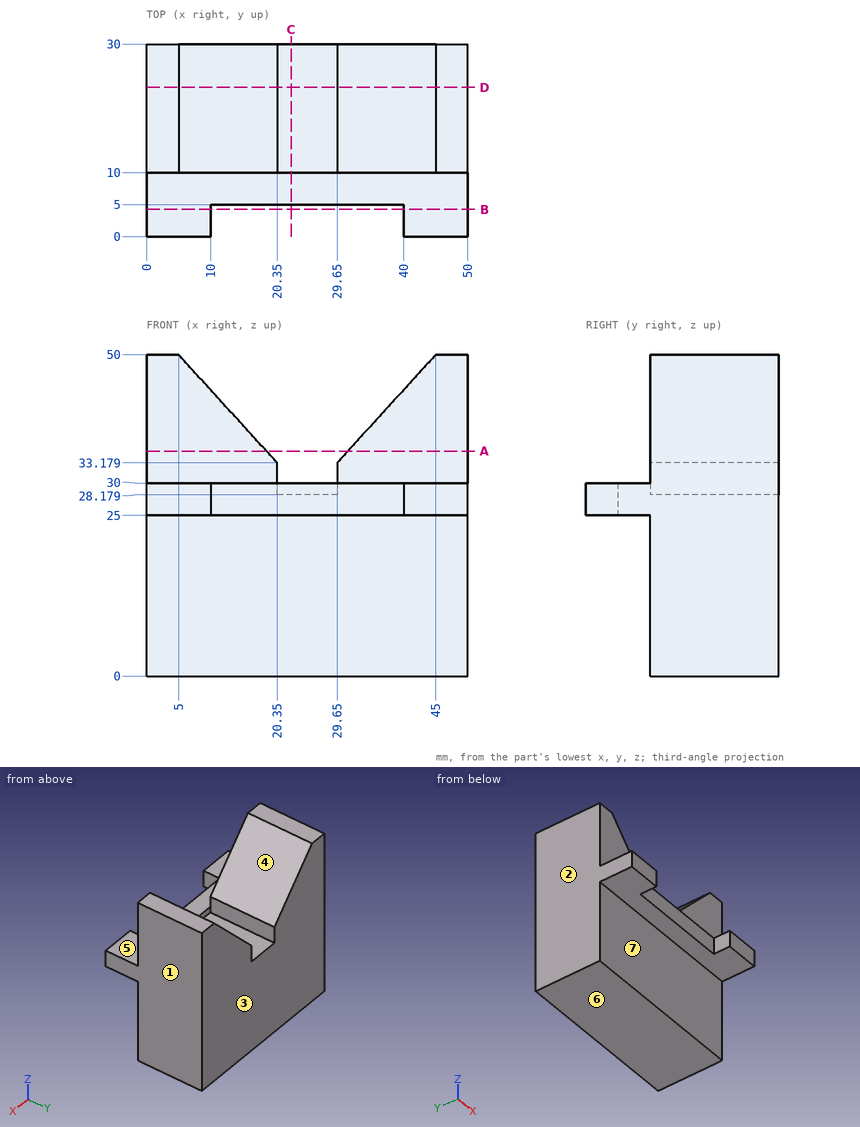
Design review of the part shown in the three views and the two pictorial views. Dimensions are in mm from the part's minimum x, y and z. A direction names the side the tool comes from. Round coordinates to 2 decimals unless told otherwise and drop trailing zeros. Loops run counter-clockwise (first coordinate to the right, second up) from the corner with the lowest first, then second, coordinate; pieces in that order, holes last. Notation, with made-up numbers: M -27.75,29.5 L -19.75,29.5 A14 cw -19.75,35.5 Z; hole C 61,-14 d4. An arc over 180 degrees is marked long. Write item = value, one per line.
Item 1: Take a section at C-C on x = 22.5. Write out the cut boundary in (y, z).
Return value:
outline = M 5,25 L 10,25 L 10,0 L 30,0 L 30,28.18 L 10,28.18 L 10,30 L 5,30 Z
Item 2: Machinability: for the marked faces 5, 6 and 7, which of the approach directions +Z, -Z, +X, -X, +Y, -Y give a long, thin tool a straight path to every point of the face, cutting with its end or side? Answer none if there is none.
Return value:
face_5 = +Z, +X, -X, -Y
face_6 = -Z, +X, -X, +Y, -Y
face_7 = -Z, +X, -X, -Y
Item 3: Take a section at D-D on y = 23.25. Write out the cut boundary in (x, z), then the cut area to 3 significant figures.
Return value:
outline = M 0,0 L 50,0 L 50,50 L 45,50 L 29.65,33.18 L 29.65,28.18 L 20.35,28.18 L 20.35,33.18 L 5,50 L 0,50 Z
area = 2,040 mm2
Item 4: Take a section at B-B on y = 4.25. Write out the cut boundary in (x, z), then the cut area to 3 significant figures.
Return value:
outline = M 0,25 L 10,25 L 10,30 L 0,30 Z; M 40,25 L 50,25 L 50,30 L 40,30 Z
area = 100 mm2
Item 5: Take a section at A-A on z = 35. Write out the cut boundary in (x, y).
Return value:
outline = M 0,10 L 18.69,10 L 18.69,30 L 0,30 Z; M 31.31,10 L 50,10 L 50,30 L 31.31,30 Z
Item 6: Insertion check: P1, Ø2.5, axis at x = 21.5, z = 28, coming from the -Y side; P2, Ø0.5, axis at x = 23, z = 29.5, coming from the +Y side; P3, Ø5, axis at x = 23, y = 5.5, coming from the -Z side; P4, Ø4, axis at y = 16.5, z = 30, coming from the -X side. Each pin has a flat end and moves straight along its axis. Give the tip position at first contact, or say it passes through.
Return value:
P1 = 5
P2 = 10
P3 = 25
P4 = 0
Item 7: The part is to be moulded in two halves that separate along X. For the marked faces 1, 2, 3 and 4, say which applies: released by +X, released by -X, zero draft, split by the parting line, or undercut.
Return value:
face_1 = released by +X
face_2 = released by -X
face_3 = zero draft
face_4 = undercut
Item 8: For line 1 (X direction, y = 22.5, z = 30.5); line 2 (Z direction, x = 2.5, y = 5.25); line 3 (Y direction, x = 19.5, z = 17), list the stretches that pass through material, from the lowest coordinate up. Write a range as [from, to].
Return value:
line_1 = [0, 20.35], [29.65, 50]
line_2 = [25, 30]
line_3 = [10, 30]
